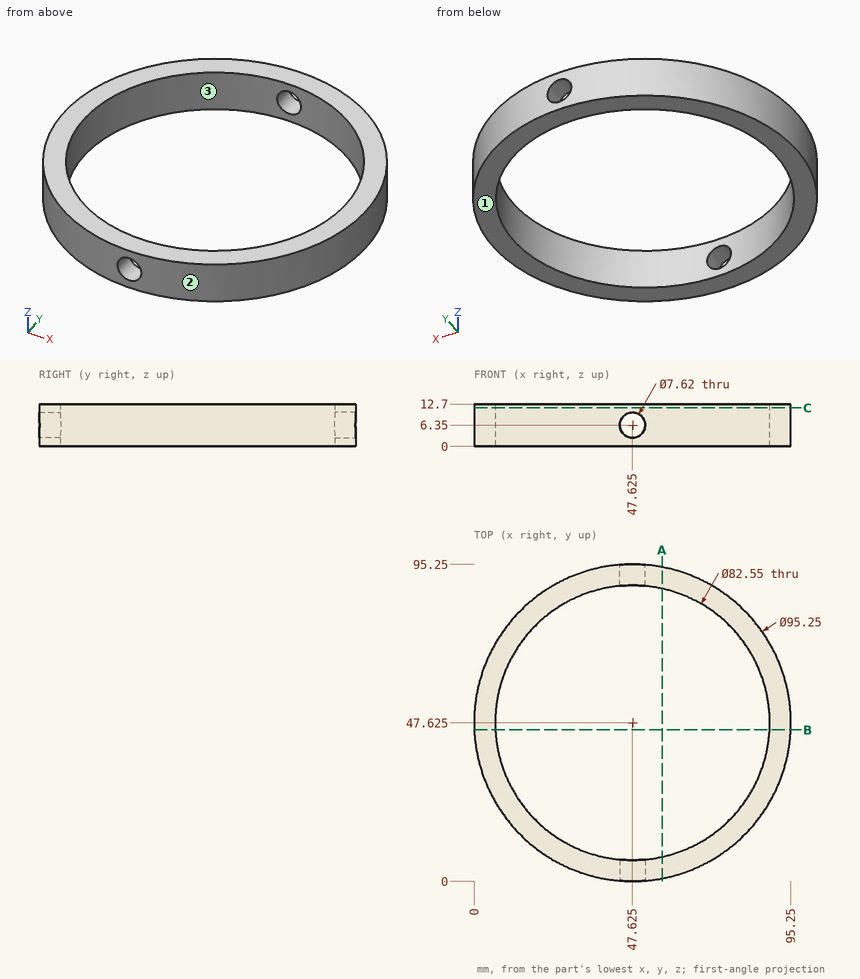
Part print with two shaded views. Sizes in mm from the minimum x, y, z corner. Coordinates: 2 decimals unless noted, no trailing zeros. Order: outer loops, then holes, each group sorted by start corner. A loop starts at its lowest first (then second) coordinate and runs counter-clockwise, first axis right, second up. Notation, with made-up numbers: (5, -18.75) - (12, -18.75) arc R14 cw to (12, -3.75) - close; hole circle Ø1 at (29.5, 56.5). An arc over 180 degrees is marked (long way). Answer in a Markdown table with one row per item.
1. Slice it at B-B, the plane y = 45.5. List the corners of the cut face in (x, z), then the cut area to 3 significant figures.
Answer:
| item | result |
|---|---|
| outline | (0.05, 0) - (6.4, 0) - (6.4, 12.7) - (0.05, 12.7) - close; (88.85, 0) - (95.2, 0) - (95.2, 12.7) - (88.85, 12.7) - close |
| area | 161 mm² |
2. Flat gauge pins, fed straight in: P1, Ø4.5, axis at x = 47.625, z = 6.35, coming from the +Y side; P2, Ø4, axis at y = 22, z = 2.5, coming from the +X side; P3, Ø1.5, axis at x = 30, z = 6.5, coming from the +Y side. Where does each tip first touch, or does it go through?
Answer:
| item | result |
|---|---|
| P1 | through |
| P2 | x = 88.98 |
| P3 | y = 92.16 |
3. Pull direction X, two halves, no side cores. Call the marked faces 1, 2 and 3: +X half, -X half, draft (parallel to the pull), parting line (faces both ways), or undercut.
Answer:
| item | result |
|---|---|
| face 1 | draft |
| face 2 | parting line |
| face 3 | undercut |
4. Slice it at C-C, the plane z = 11.5. List the corners of the cut face in (x, y) (3 decimals), then the cut area to 3 significant figures.
Answer:
| item | result |
|---|---|
| outline | circle Ø95.25 at (47.625, 47.625); hole circle Ø82.55 at (47.625, 47.625) |
| area | 1,770 mm² |
5. Slice it at A-A, the plane x = 56.5. List the corners of the cut face in (y, z).
Answer:
| item | result |
|---|---|
| outline | (0.83, 0) - (7.32, 0) - (7.32, 12.7) - (0.83, 12.7) - close; (87.93, 0) - (94.42, 0) - (94.42, 12.7) - (87.93, 12.7) - close |
6. Drill centre lines: L1, parallel to Y at x = 64, z = 11; L2, parallel to Y at x = 9.5, z = 12; L3, parallel to X at y = 33, z = 7.5. Where is each one in solid material? Low to high. Write a range as from..to.
Answer:
| item | result |
|---|---|
| L1 | 2.9..9.74, 85.51..92.35 |
| L2 | 19.08..31.81, 63.44..76.17 |
| L3 | 2.3..9.03, 86.22..92.95 |
